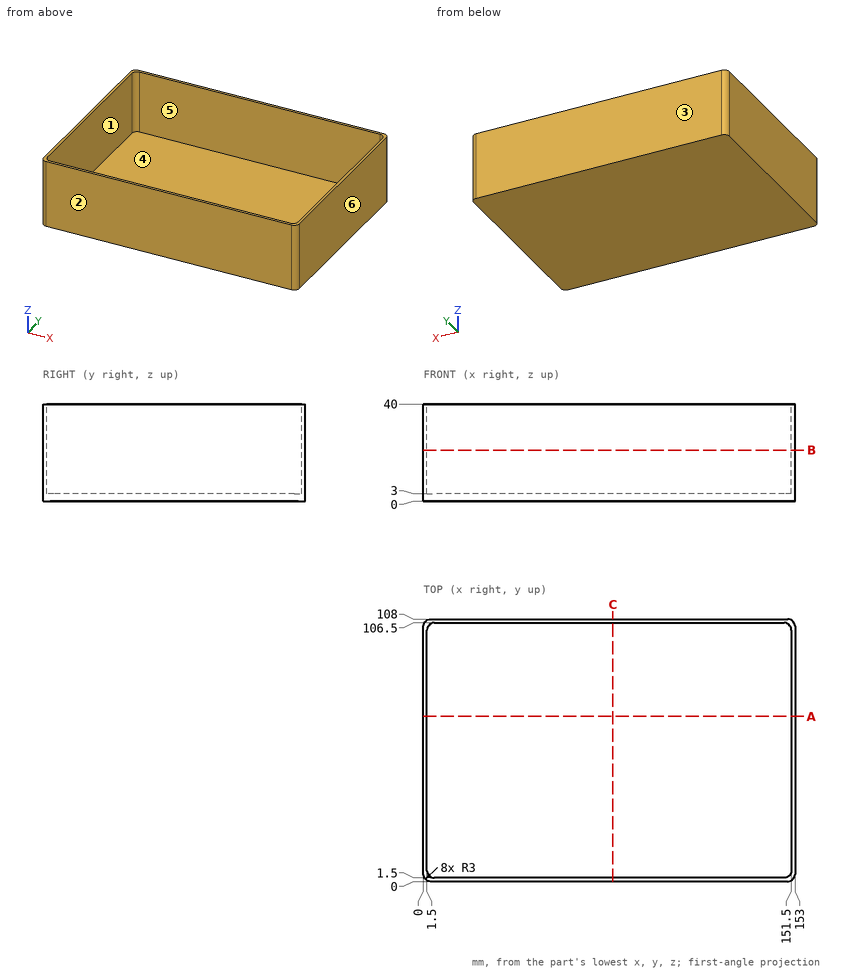
Here's the drawing with two shaded views (mm, measured from the low corner). I have some questions. A direction names the side the tool comes from. Coordinates: 2 decimals unless noted, no trailing zeros. Write each loop counter-clockwise with the first axis right and the second up, starting at its lowest first coordinate (ties: lowest second). Pieces come first, ordered by that corner, then holes. Notation, with made-up numbers: M -30,0.25 L -26,0.25 A26 cw -26,20.25 Z; hole C 4,77 d10. An arc over 180 degrees is marked long. Use one line per item in the form item = value.
Q1. For the marked faces 5 and 6, which set-ups out of +Z, -Z, +X, -X, +Y, -Y let a thin tool reach every point of the face, with its end or its side?
Model answer:
face_5 = +Z
face_6 = +Z, -Z, +X, +Y, -Y
Q2. If we section it at C-C (x = 78): Write out the boundary of the cut face in (y, z).
Model answer:
outline = M 0,0 L 108,0 L 108,40 L 106.5,40 L 106.5,3 L 1.5,3 L 1.5,40 L 0,40 Z
Q3. I need wall thicknesses on line 1 along X through (y, z) = (53, 33); line 2 along Y through (x, z) = (89, 9); line 3 along Z through (x, y) = (138.5, 59.5). Which ranges of each line are inside material? Lowest first, please. Write a range as from..to.
Model answer:
line_1 = 0..1.5, 151.5..153
line_2 = 0..1.5, 106.5..108
line_3 = 0..3
Q4. If we section it at B-B (z = 21): Write out the boundary of the cut face in (x, y).
Model answer:
outline = M 0,3 A3 ccw 3,0 L 150,0 A3 ccw 153,3 L 153,105 A3 ccw 150,108 L 3,108 A3 ccw 0,105 Z; hole M 1.5,4.5 A3 ccw 4.5,1.5 L 148.5,1.5 A3 ccw 151.5,4.5 L 151.5,103.5 A3 ccw 148.5,106.5 L 4.5,106.5 A3 ccw 1.5,103.5 Z
Q5. For P1, Ø10, axis at x = 119.5, z = 24, coming from the -Y side; P2, Ø4, axis at x = 111.5, y = 32, coming from the +Z side, each with a flat end and sliding along its axis, tell me the tip position at first contact or that it passes through.
Model answer:
P1 = 0
P2 = 3
Q6. If we section it at A-A (y = 68): Write out the boundary of the cut face in (x, z).
Model answer:
outline = M 0,0 L 153,0 L 153,40 L 151.5,40 L 151.5,3 L 1.5,3 L 1.5,40 L 0,40 Z
Q7. We'd pull the mould along Y, two halves only. Please class the marked faces 1, 2, 3 and 4: +Y half, -Y half, draft (parallel to the pull), parting line (faces both ways), or undercut.
Model answer:
face_1 = undercut
face_2 = -Y half
face_3 = +Y half
face_4 = undercut
